Geometry check sheet. Reference: drawing and pictorial views, mm from the part's lowest x, y, z. A direction names the side the tool comes from. Give positions to 0.01 mm unless a question says otherwise; leave off trailing zeros. Write each loop counter-clockwise with the first axis right and the second up, starting at its lowest first coordinate (ties: lowest second). Pieces come first, ordered by that corner, then holes. Notation, with made-up numbers: (35.5, -13.75) - (71.5, -13.75) arc R30 cw to (71.5, 24.25) - close; hole circle Ø7 at (-39.75, -24). An arc over 180 degrees is marked (long way). Put each result on its own line as item: value.
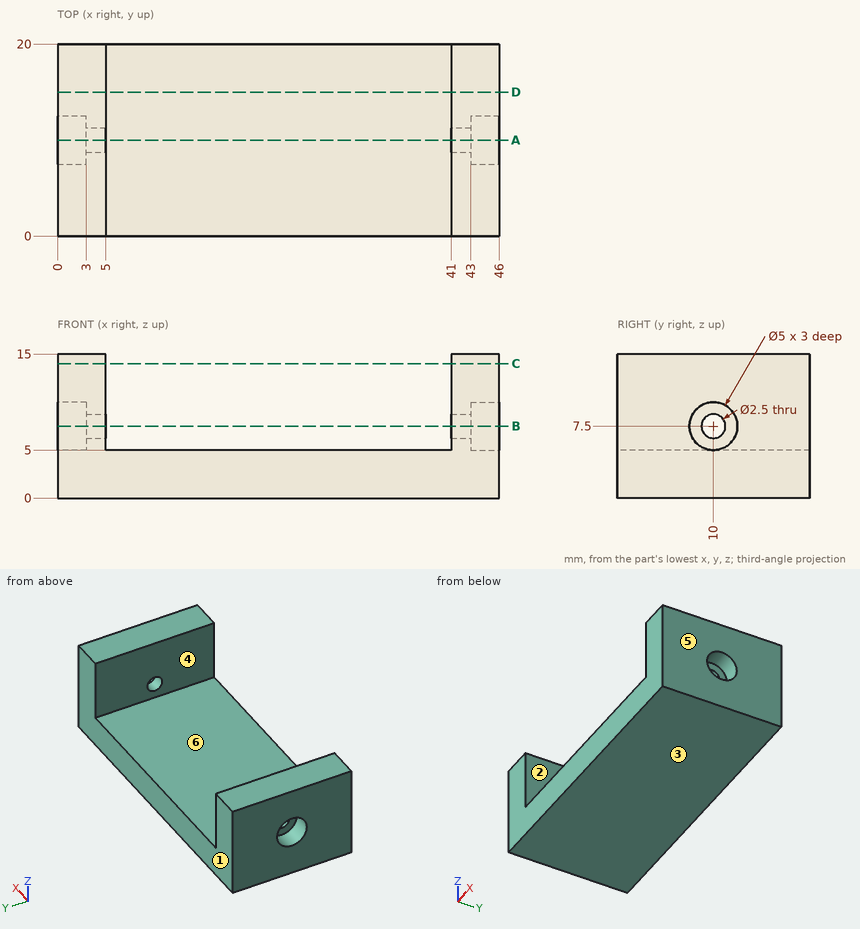
Q1. Release check for a two-part mould opening along X. For the marked faces 3, 4, 5 and 6 record: released by +X, released by -X, zero draft, split by the parting line, or undercut.
Answers follow:
face 3: zero draft
face 4: undercut
face 5: released by +X
face 6: undercut
Q2. Section check D-D, the plane y = 15. Record the cut outline in (x, z).
Answers follow:
outline: (0, 0) - (46, 0) - (46, 15) - (41, 15) - (41, 5) - (5, 5) - (5, 15) - (0, 15) - close
Q3. Scan lines: line 1 along X through (y, z) = (13.25, 6.75); line 2 along Z through (x, y) = (2, 10); line 3 along Z through (x, y) = (42.3, 10). Record each from-to range of solid material in increasing order.
Answers follow:
line 1: x = 0 to 5, 41 to 46
line 2: z = 0 to 5, 10 to 15
line 3: z = 0 to 6.25, 8.75 to 15
Q4. Section check B-B, the plane z = 7.5. Record the cut outline in (x, y), plus the area to 3 significant figures.
Answers follow:
outline: (0, 0) - (5, 0) - (5, 8.75) - (3, 8.75) - (3, 7.5) - (0, 7.5) - close; (0, 12.5) - (3, 12.5) - (3, 11.25) - (5, 11.25) - (5, 20) - (0, 20) - close; (41, 0) - (46, 0) - (46, 7.5) - (43, 7.5) - (43, 8.75) - (41, 8.75) - close; (41, 11.25) - (43, 11.25) - (43, 12.5) - (46, 12.5) - (46, 20) - (41, 20) - close
area: 160 mm2
Q5. Go/stop test with flat-tipped pins: pin 1 Ø2 at (y, z) = (10, 7.5) entering from -X; pin 2 Ø3 at (y, z) = (10, 7.5) entering from -X; pin 3 Ø10 at (x, y) = (22, 5.5) entering from +Z; pin 4 Ø5.5 at (y, z) = (9.5, 8.5) entering from -X. Record where each tip stops, or that it passes through.
Answers follow:
pin 1: passes through
pin 2: stops at x = 3
pin 3: stops at z = 5
pin 4: stops at x = 0
Q6. Section check A-A, the plane y = 10. Record the cut outline in (x, z), plus the area to 3 significant figures.
Answers follow:
outline: (0, 0) - (46, 0) - (46, 5) - (43, 5) - (43, 6.25) - (41, 6.25) - (41, 5) - (5, 5) - (5, 6.25) - (3, 6.25) - (3, 5) - (0, 5) - close; (0, 10) - (3, 10) - (3, 8.75) - (5, 8.75) - (5, 15) - (0, 15) - close; (41, 8.75) - (43, 8.75) - (43, 10) - (46, 10) - (46, 15) - (41, 15) - close
area: 290 mm2
Q7. Section check C-C, the plane z = 14. Record the cut outline in (x, y).
Answers follow:
outline: (0, 0) - (5, 0) - (5, 20) - (0, 20) - close; (41, 0) - (46, 0) - (46, 20) - (41, 20) - close
Q8. Set-up check for the marked faces 1 and 2: record each of +Z, -Z, +X, -X, +Y, -Y from which the full face is reachable in a straight line by a thin tool's end or side.
Answers follow:
face 1: +Z, -Z, +X, -X, +Y
face 2: +Z, +Y, -Y
